Input: part model. Units: mm. Frame: model coordinates. A direction names the side the tool comes from. Round coordinates to 2 decimals unless told otherwise and drop trailing zeros. Write each loop counter-clockwise with the first axis right and the second up, starting at its lowest first coordinate (ties: lowest second). Pieces come first, ordered by that corner, then holes. Notation, with made-up numbers: M 36,-26 L 73,-26 A12 ccw 73,-3 Z; hole C 2,20 d7. An arc over 180 degrees is marked long. Use one line per item in the form item = value. Start each with the question number.
```python
from build123d import *

# Parameters (mm, degrees)
SKETCH1_R           = 8
SKETCH1_R_2         = 2.5
BOSS_EXTRUDE1_DEPTH = 23
SKETCH2_W           = 12.136901607
SKETCH2_H           = 1.2
SKETCH2_W_2         = 11.75463699
CUT_EXTRUDE1_DEPTH  = 9
CIRPATTERN1_COUNT   = 2
SKETCH3_W           = 1.2
SKETCH3_H           = 8.369278369
SKETCH3_H_2         = 8.338508964
SKETCH3_H_3         = 7.969276094
CUT_EXTRUDE2_DEPTH  = 9
CIRPATTERN2_COUNT   = 2


with BuildPart() as part:
    # Sketch1 → Boss-Extrude1 (new body)
    with BuildSketch(Plane.XY):
        Circle(SKETCH1_R)
        Circle(SKETCH1_R_2, mode=Mode.SUBTRACT)
    extrude(amount=BOSS_EXTRUDE1_DEPTH)

    # Sketch2 → Cut-Extrude1 (cut, symmetric)
    with BuildSketch(Plane(origin=(0, 0, 0), x_dir=(1, 0, 0), z_dir=(0, 1, 0))):
        with Locations((-9.068450803, -7.616722674)):
            Rectangle(SKETCH2_W, SKETCH2_H)
        with Locations((-8.877318495, -14.571215167)):
            Rectangle(SKETCH2_W_2, SKETCH2_H)
    cut_extrude1 = extrude(amount=CUT_EXTRUDE1_DEPTH, both=True, mode=Mode.SUBTRACT)

    # CirPattern1: Cut-Extrude1 ×2 about axis
    cirpattern1_axis = Axis((0, 0, 23), (0, 0, -1))
    for i in range(1, CIRPATTERN1_COUNT):
        add(cut_extrude1.rotate(cirpattern1_axis, i * 360 / CIRPATTERN1_COUNT), mode=Mode.SUBTRACT)

    # Sketch3 → Cut-Extrude2 (cut, symmetric)
    with BuildSketch(Plane(origin=(0, 0, 0), x_dir=(0, 0, -1), z_dir=(1, 0, 0))):
        with Locations((-11.201145593, 7.184639184)):
            Rectangle(SKETCH3_W, SKETCH3_H)
        with Locations((-17.65104418, 7.169254482)):
            Rectangle(SKETCH3_W, SKETCH3_H_2)
        with Locations((-4.751247006, 6.984638047)):
            Rectangle(SKETCH3_W, SKETCH3_H_3)
    cut_extrude2 = extrude(amount=CUT_EXTRUDE2_DEPTH, both=True, mode=Mode.SUBTRACT)

    # CirPattern2: Cut-Extrude2 ×2 about axis
    cirpattern2_axis = Axis((0, 0, 23), (0, 0, -1))
    for i in range(1, CIRPATTERN2_COUNT):
        add(cut_extrude2.rotate(cirpattern2_axis, i * 360 / CIRPATTERN2_COUNT), mode=Mode.SUBTRACT)


solid = part.part
```
Item 1: Ray query, line 1 (Z direction, x = 2, y = -4.5); line 2 (Z direction, x = -4, y = 0.75); line 3 (Y direction, x = 0, z = 5). Return the intervals inside material, ascending. Write a range as from..to.
Item 2: Cut plane D-D (y = 2). Output: boundary loops of the cut face in (x, z), plus the area to 3 significant figures.
Item 3: Reachability of faces 4 (the face through (0, 5, 18.251)), 5 (the face through (3, 0, 8)), 6 (the face through (-5, 0, 8.217)) from +Z, -Z, +X, -X, +Y, -Y: full face, straight path, thin tool, end or side. Return the list, or none.
Item 4: Cut plane C-C (z = 14.5). Output: boundary loops of the cut face in (x, y).
Item 5: First-contact query: pin 1 (1.3 mm diameter, centred on x = 1, z = 18, fed in from -Y); pin 2 (4 mm diameter, centred on y = 4.5, z = 5.5, fed in from +X); pin 3 (0.6 mm diameter, centred on x = 0.5, z = 18, fed in from +Y). Flat tips, straight axial feed; report the tip coordinate or a pass-through.
Item 6: Cut plane A-A (y = 0). Output: boundary loops of the cut face in (x, z).
Item 7: Draft query along Z for faces 1 (the face through (2, 2, 0)), 2 (the face through (2, 2, 23)), 3 (the face through (3, 0, 15)). Return one class per face: +Z half, -Z half, draft (parallel to the pull), parting line (faces both ways), or undercut.
Final values:
q1.line_1 = 0..4.15, 5.35..10.6, 11.8..17.05, 18.25..23
q1.line_2 = 0..7.02, 8.22..13.97, 15.17..23
q1.line_3 = -3..-2.5, 2.5..3
q2.outline = M -7.75,0 L -1.5,0 L -1.5,23 L -7.75,23 L -7.75,15.17 L -3,15.17 L -3,13.97 L -7.75,13.97 L -7.75,8.22 L -3,8.22 L -3,7.02 L -7.75,7.02 Z; M 1.5,0 L 7.75,0 L 7.75,7.02 L 3,7.02 L 3,8.22 L 7.75,8.22 L 7.75,13.97 L 3,13.97 L 3,15.17 L 7.75,15.17 L 7.75,23 L 1.5,23 Z
q2.area = 265 mm^2
q3.face_4 = +X, -X, +Y
q3.face_5 = +X, +Y, -Y
q3.face_6 = -X, +Y, -Y
q4.outline = M -3,-7.42 A8 ccw 3,-7.42 L 3,7.42 A8 ccw -3,7.42 Z; hole C 0,0 d5
q5.pin_1 = -7.99
q5.pin_2 = 7.6
q5.pin_3 = 7.99
q6.outline = M -8,0 L -2.5,0 L -2.5,23 L -8,23 L -8,15.17 L -3,15.17 L -3,13.97 L -8,13.97 L -8,8.22 L -3,8.22 L -3,7.02 L -8,7.02 Z; M 2.5,0 L 8,0 L 8,7.02 L 3,7.02 L 3,8.22 L 8,8.22 L 8,13.97 L 3,13.97 L 3,15.17 L 8,15.17 L 8,23 L 2.5,23 Z
q7.face_1 = -Z half
q7.face_2 = +Z half
q7.face_3 = undercut
